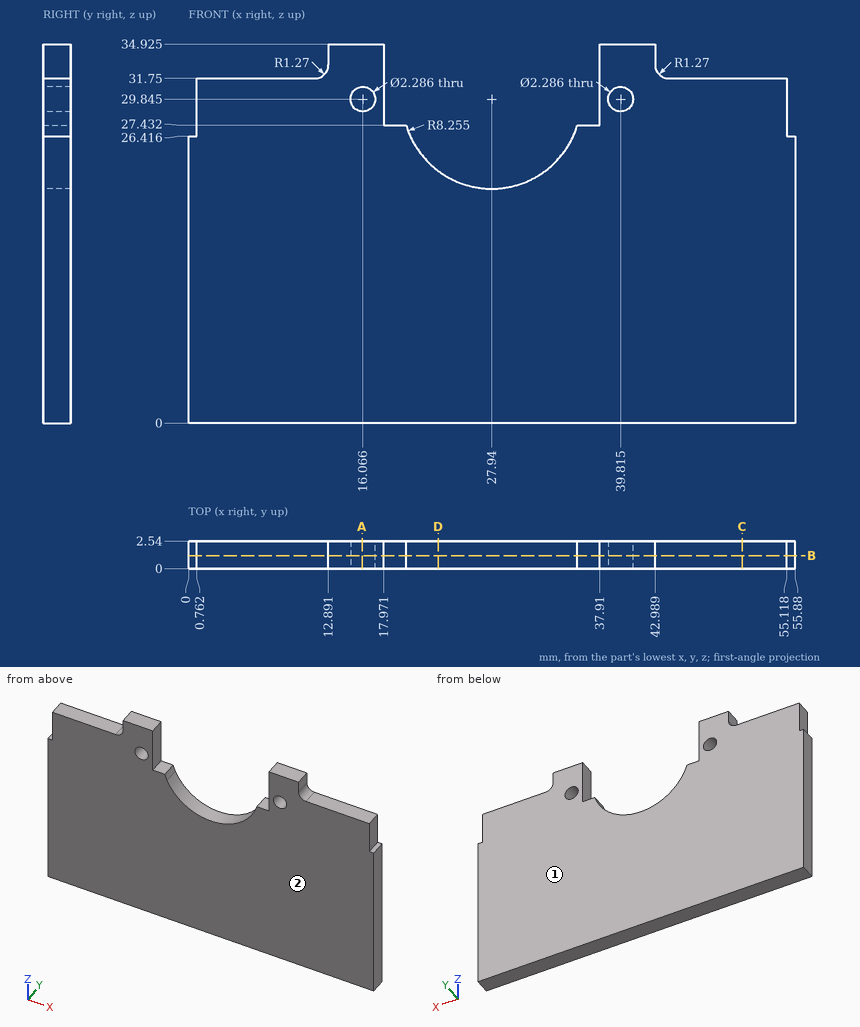
Source: three-view drawing plus pictorial views. Frame: mm from the lowest corner of the part. Round coordinates to 2 decimals unless told otherwise and drop trailing zeros. Loops run counter-clockwise (first coordinate to the right, second up) from the corner with the lowest first, then second, coordinate; pieces in that order, holes last.
1. Section query D-D on x = 23. Output: boundary loops of the cut face in (y, z).
2. Contact query for flat-ended pins moving along their axis: pin 1 (0.8 mm diameter, centred on x = 51.5, y = 1, fed in from +Z); pin 2 (1.5 mm diameter, centred on y = 1, z = 34.5, fed in from -X); pin 3 (0.6 mm diameter, centred on x = 55.5, y = 1.5, fed in from +Z). Output: stop coordinate, or through.
3. Section query A-A on x = 16. Output: boundary loops of the cut face in (y, z) (1 decimal).
4. Mould query, pull axis Y, two halves, no side actions, for the marked faces 1 and 2. Classes: released by +Y, released by -Y, zero draft, split by the parting line, or undercut.
5. Section query B-B on y = 1.2. Give the number of separate pieces and of enclosed holes in the cut face, and give its area (3 significant figures).
6. Section query C-C on x = 51. Output: boundary loops of the cut face in (y, z).
7. Ray query, L1, parallel to X at y = 1.8, z = 30; L2, parallel to X at y = 0.4, z = 27.5; L3, parallel to X at y = 1.1, z = 29 (1 decimal). Return the intervals inside material, ascending.
Answers below:
1. outline: (0, 0) - (2.54, 0) - (2.54, 23.23) - (0, 23.23) - close
2. pin 1: stops at z = 31.75
2. pin 2: stops at x = 12.89
2. pin 3: stops at z = 26.42
3. outline: (0, 0) - (2.5, 0) - (2.5, 28.7) - (0, 28.7) - close; (0, 31) - (2.5, 31) - (2.5, 34.9) - (0, 34.9) - close
4. face 1: released by +Y
4. face 2: released by -Y
5. separate pieces: 1
5. enclosed holes: 2
5. area: 1,640 mm2
6. outline: (0, 0) - (2.54, 0) - (2.54, 31.75) - (0, 31.75) - close
7. L1: x = 0.76 to 14.93, 17.2 to 17.97, 37.91 to 38.68, 40.95 to 55.12
7. L2: x = 0.76 to 17.97, 37.91 to 55.12
7. L3: x = 0.8 to 15.3, 16.8 to 18, 37.9 to 39, 40.6 to 55.1
